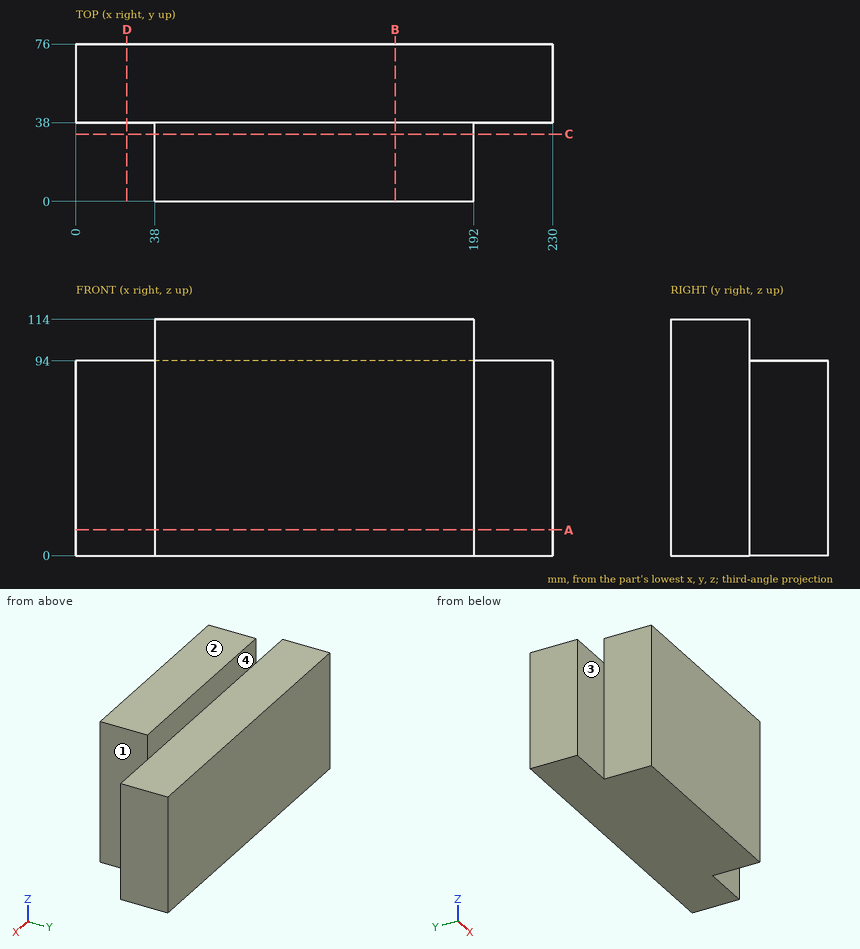
Answer from the drawing. Dimensions are ordinates in mm from the lowest x, y and z of the part. A direction names the side the tool comes from. Coordinates: 2 decimals unless noted, no trailing zeros. Write each loop counter-clockwise with the first axis right and the second up, starting at its lowest first coordinate (ties: lowest second). Pieces come first, ordered by that corner, then holes. Notation, with made-up numbers: M 7.25,-25 L 30.25,-25 A25 ccw 30.25,6 Z; hole C 78,-39 d3. An arc over 180 degrees is marked long. Write item = value, one per line.
1. For the marked faces 1, 2, 3 and 4, determine the directions among +Z, -Z, +X, -X, +Y, -Y from which every point of the face is accessible in a straight line to the end or side of a thin tool.
Solution:
face_1 = +Z, -Z, +X, -Y
face_2 = +Z, +X, -X, +Y, -Y
face_3 = +Z, -Z, -X, -Y
face_4 = +Z, +X, -X, +Y
2. Straight lines are drawn through the part: line 1 (Z direction, x = 13.5, y = 65); line 2 (Y direction, x = 14, z = 17); line 3 (X direction, y = 27, z = 62.5). For each, find the intervals that lie inside material, in ascending order. Write a range as from..to.
Solution:
line_1 = 0..94
line_2 = 38..76
line_3 = 38..192
3. Flat-ended cylindrical pins translate along their axes: pin 1 (10 mm diameter, centred on x = 110, y = 57.5, fed in from -Z); pin 2 (11.5 mm diameter, centred on y = 17, z = 82, fed in from +X); pin 3 (19 mm diameter, centred on x = 78.5, y = 49, fed in from +Z); pin 4 (11.5 mm diameter, centred on y = 22, z = 79, fed in from -X). Find the tip coordinate at first contact, or state that the pin passes through.
Solution:
pin_1 = 0
pin_2 = 192
pin_3 = 94
pin_4 = 38
4. The part is cut by section D-D (x = 24.5). Determine the outline of the cut face in (y, z).
Solution:
outline = M 38,0 L 76,0 L 76,94 L 38,94 Z
5. The part is cut by section B-B (x = 154). Determine the outline of the cut face in (y, z), then the cut area to 3 significant figures.
Solution:
outline = M 0,0 L 76,0 L 76,94 L 38,94 L 38,114 L 0,114 Z
area = 7,900 mm2
6. The part is cut by section A-A (z = 12.5). Determine the outline of the cut face in (x, y).
Solution:
outline = M 0,38 L 38,38 L 38,0 L 192,0 L 192,38 L 230,38 L 230,76 L 0,76 Z
7. The part is cut by section C-C (y = 32.5). Determine the outline of the cut face in (x, z), then the cut area to 3 significant figures.
Solution:
outline = M 38,0 L 192,0 L 192,114 L 38,114 Z
area = 17,600 mm2
